from build123d import *

# Parameters (mm, degrees)
EXTRUDE_1_DEPTH = 48
FILLET_2_R      = 10
FILLET_3_R      = 10


with BuildPart() as part:
    # 草图1 → 凸台-拉伸1 (new body)
    with BuildSketch(Plane.XY):
        with BuildLine():
            Line((-50, 50), (-50, -50))
            Line((-50, -50), (0, -50))
            Line((0, -50), (0, -20.9))
            ThreePointArc((0, -20.9), (-20.9, 0), (0, 20.9))
            Line((0, 20.9), (0, 50))
            Line((0, 50), (-50, 50))
        make_face()
        with BuildLine():
            Line((50, 50), (0, 50))
            Line((0, 50), (0, 20.9))
            ThreePointArc((0, 20.9), (14.778531727, 14.778531727), (20.9, 0))
            Line((20.9, 0), (50, 0))
            Line((50, 0), (50, 50))
        make_face()
        with BuildLine():
            Line((0, -13.339839146), (0, -20.9))
            ThreePointArc((0, -20.9), (14.778531727, -14.778531727), (20.9, 0))
            Line((20.9, 0), (13.339839146, 0))
            ThreePointArc((13.339839146, 0), (9.43269072, -9.43269072), (0, -13.339839146))
        make_face()
        with BuildLine():
            ThreePointArc((20.9, 0), (14.778531727, 14.778531727), (0, 20.9))
            Line((0, 20.9), (0, 13.339839146))
            ThreePointArc((0, 13.339839146), (9.43269072, 9.43269072), (13.339839146, 0))
            Line((13.339839146, 0), (20.9, 0))
        make_face()
        with BuildLine():
            ThreePointArc((0, 20.9), (-20.9, 0), (0, -20.9))
            Line((0, -20.9), (0, -13.339839146))
            ThreePointArc((0, -13.339839146), (-13.339839146, 0), (0, 13.339839146))
            Line((0, 13.339839146), (0, 20.9))
        make_face()
        with BuildLine():
            Line((0, -20.9), (0, -50))
            Line((0, -50), (50, -50))
            Line((50, -50), (50, 0))
            Line((50, 0), (20.9, 0))
            ThreePointArc((20.9, 0), (14.778531727, -14.778531727), (0, -20.9))
        make_face()
    extrude(amount=EXTRUDE_1_DEPTH)

    # 圆角2
    fillet_2_edges = [part.edges().sort_by_distance(p)[0] for p in [
        (50, -50, 24),
        (-50, -50, 24),
        (-50, 50, 24),
        (50, 50, 24),
    ]]
    fillet(fillet_2_edges, radius=FILLET_2_R)

    # 圆角3
    fillet_3_edges = [part.edges().sort_by_distance(p)[0] for p in [
        (0, -50, 48),
        (-50, 0, 48),
        (50, 0, 48),
        (0, 50, 48),
        (-47.071067812, 47.071067812, 48),
        (47.071067812, 47.071067812, 48),
        (47.071067812, -47.071067812, 48),
        (-47.071067812, -47.071067812, 48),
    ]]
    fillet(fillet_3_edges, radius=FILLET_3_R)


solid = part.part
Verification items for the finished model (mm, model axes). Round coordinates to 2 decimals unless told otherwise and drop trailing zeros. Order: outer loops, then holes, each group sorted by start corner. A loop starts at its lowest first (then second) coordinate and runs counter-clockwise, first axis right, second up. Notation, with made-up numbers: (12.25, 29.5) -> (45.25, 29.5) arc R8 ccw to (45.25, 44.5) -> close; hole circle Ø2 at (31.5, 55). An arc over 180 degrees is marked (long way). Put each result on its own line as item: value.
1) Material ranges on line 1 (Y direction, x = 10.5, z = 16.5); line 2 (Y direction, x = 7, z = 43.5); line 3 (X direction, y = -11, z = 41), recorded low to high.
Final values:
line 1: y = -50 to -8.23, 8.23 to 50
line 2: y = -48.35 to -11.36, 11.36 to 48.35
line 3: x = -49.54 to -7.55, 7.55 to 49.54
2) Mould release check, pull along Z, two halves, no side actions. Record for faces 1 (the flat face through (-12, 12, 0)), 2 (the flat face through (-1, 18, 48)), 3 (the flat face through (-50, 1, 19)): +Z half, -Z half, draft (parallel to the pull), parting line (faces both ways), or undercut.
Final values:
face 1: -Z half
face 2: +Z half
face 3: draft
3) Section check C-C (y = 5). Record the cut outline in (x, z), then the cut area to 3 significant figures.
Final values:
outline: (-50, 0) -> (-12.37, 0) -> (-12.37, 48) -> (-40, 48) arc R10 ccw to (-50, 38) -> close; (12.37, 0) -> (50, 0) -> (50, 38) arc R10 ccw to (40, 48) -> (12.37, 48) -> close
area: 3,570 mm^2
4) Section check B-B (z = 36.5). Record the cut outline in (x, y), then the cut area to 3 significant figures.
Final values:
outline: (-50, -40) arc R10 ccw to (-40, -50) -> (40, -50) arc R10 ccw to (50, -40) -> (50, 40) arc R10 ccw to (40, 50) -> (-40, 50) arc R10 ccw to (-50, 40) -> close; hole circle Ø26.68 at (0, 0)
area: 9,360 mm^2
5) Section check A-A (y = -10). Record the cut outline in (x, z), then the cut area to 3 significant figures.
Final values:
outline: (-50, 0) -> (-8.83, 0) -> (-8.83, 48) -> (-40, 48) arc R10 ccw to (-50, 38) -> close; (8.83, 0) -> (50, 0) -> (50, 38) arc R10 ccw to (40, 48) -> (8.83, 48) -> close
area: 3,910 mm^2
